Check sheet for the modelled part. Datum: model origin and axes. Units: mm. Face numbers are marked on the shaded views. A direction names the side the tool comes from. Coordinates: 2 decimals unless noted, no trailing zeros. Loops run counter-clockwise (first coordinate to the right, second up) from the corner with the lowest first, then second, coordinate; pieces in that order, holes last. Notation, with made-up numbers: (14, -9.5) -> (33, -9.5) arc R12 cw to (33, 7.5) -> close; hole circle Ø3 at (10.25, 54.5). An arc over 180 degrees is marked (long way). Use CSV: the item, a comma, the result in double quotes. Start each with the question number.
1. Sectioned sample at D-D, the plane y = -29. Record the cut outline in (x, z), and give its area (3 significant figures).
2. Sectioned sample at A-A, the plane z = 33. Record the cut outline in (x, y), and give its area (3 significant figures).
3. Set-up check for the marked faces 5, 6, 7 and 8: record each of +Z, -Z, +X, -X, +Y, -Y from which the full face is reachable in a straight line by a thin tool's end or side.
4. Release check for a two-part mould opening along X. For the marked faces 1, 2, 3 and 4 record: pulls with the +X half, pulls with the -X half, needs draft (parallel to the pull), parting line crosses it, or undercut.
5. Sectioned sample at C-C, the plane y = 0. Record the cut outline in (x, z).
6. Thickness scan on L1, parallel to Y at x = 10.5, z = 58; L2, parallel to Z at x = 53, y = -36.5; L3, parallel to Z at x = -14, y = -25.5. Record the ranges inside material, lowest first.
7. Gauge pin test, flat ends, axial feed: pin 1 (5 mm diameter, centred on x = -14.5, z = 63.5, fed in from +Y); pin 2 (16.5 mm diameter, centred on y = 27, z = 24.5, fed in from -X); pin 3 (6 mm diameter, centred on x = 31.5, z = 44.5, fed in from +Y); pin 4 (16 mm diameter, centred on x = 45.12, y = 0.47, fed in from +Z). Record the tip position at first contact, or that the pin passes through.
8. Sectioned sample at B-B, the plane x = 82. Record the cut outline in (y, z).
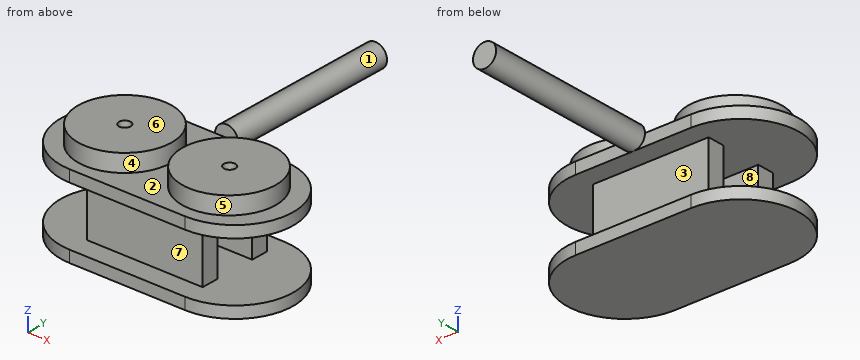
Autodesk Inventor part; units mm, degrees
ref_plane "YZ Plane" through (0, 0, 0) normal (1, 0, 0) x (0, 1, 0)
ref_plane "XZ Plane" through (0, 0, 0) normal (0, 1, 0) x (-1, 0, 0)
ref_plane "XY Plane" through (0, 0, 0) normal (0, 0, 1) x (1, 0, 0)
sketch "Sketch24" plane through (0, 0, 0) normal (0, 0, 1) x (1, 0, 0)
  line L0 (50, -50) -> (-50, -50)
  line L1 (-50, -50) -> (-50, 50)
  line L2 (-50, 50) -> (50, 50)
  line L3 (50, 50) -> (50, -50)
  line L4 (50, -50) -> (-50, 50) construction
  line L5 (-50, -50) -> (50, 50) construction
  circle A0 centre (50, 0) radius 50
  circle A1 centre (-50, 0) radius 50
  point P0 (0, 0)
  dimension "d55" = 100
  dimension "d56" = 100
  dimension "d57" = 100
  dimension "d58" = 100
extrude "Extrusion9" add sketch "Sketch24" along normal blind 10
sketch "Sketch25" plane through (0, 0, 10) normal (0, 0, 1) x (1, 0, 0)
  line L0 (50, 32.5) -> (-50, 32.5)
  line L1 (-50, 32.5) -> (-50, 17.5)
  line L2 (-50, 17.5) -> (50, 17.5)
  line L3 (50, 17.5) -> (50, 32.5)
  line L4 (50, 32.5) -> (-50, 17.5) construction
  line L5 (-50, 32.5) -> (50, 17.5) construction
  line L6 (50, -32.5) -> (-50, -32.5)
  line L7 (-50, -32.5) -> (-50, -17.5)
  line L8 (-50, -17.5) -> (50, -17.5)
  line L9 (50, -17.5) -> (50, -32.5)
  line L10 (50, -32.5) -> (-50, -17.5) construction
  line L11 (-50, -32.5) -> (50, -17.5) construction
  point P0 (0, 0)
  point P1 (0, 25)
  point P2 (0, -25)
  dimension "d61" = 100
  dimension "d62" = 15
  dimension "d63" = 15
extrude "Extrusion10" add sketch "Sketch25" along normal blind 50
sketch "Sketch38" plane through (0, 0, 60) normal (0, 0, 1) x (1, 0, 0)
  point P0 (0, 0)
sketch "Sketch39" plane through (0, 0, 10) normal (0, 0, 1) x (1, 0, 0)
  line L0 (-50, 17.5) -> (50, 17.5)
  point P0 (0, 0)
  dimension "d78" = 17.5
sketch "Sketch40" plane through (0, 0, 60) normal (0, 0, 1) x (1, 0, 0)
  line L0 (50, 50) -> (-50, 50)
  line L1 (-50, 50) -> (-50, -50)
  line L2 (-50, -50) -> (50, -50)
  line L3 (50, -50) -> (50, 50)
  line L4 (50, 50) -> (-50, -50) construction
  line L5 (-50, 50) -> (50, -50) construction
  circle A0 centre (50, 0) radius 50
  circle A1 centre (-50, 0) radius 50
  point P0 (0, 0)
  dimension "d79" = 100
  dimension "d80" = 100
  dimension "d81" = 100
  dimension "d82" = 100
extrude "Extrusion12" add sketch "Sketch40" along normal blind 10
sketch "Sketch43" plane through (0, 0, 70) normal (0, 0, 1) x (1, 0, 0)
  circle A0 centre (45, 0) radius 40
  circle A1 centre (-45, 0) radius 40
  point P0 (0, 0)
  dimension "d87" = 80
  dimension "d88" = 80
extrude "Extrusion13" add sketch "Sketch43" along normal blind 15
thread "Thread1"
thread "Thread2"
sketch "Sketch44" plane through (-45, 0, 85) normal (0, 0, 1) x (1, 0, 0)
  point P0 (45, 0)
  point P1 (0.1207, -0.2375)
hole "Hole1" at (-44.8793, -0.2375, 85) direction (0, 0, -1) diameter 10 depth 15
sketch "Sketch45" plane through (45, 0, 85) normal (0, 0, 1) x (1, 0, 0)
  point P0 (-45, 0)
  point P1 (0.1167, 0.4749)
hole "Hole2" at (45.1167, 0.4749, 85) direction (0, 0, -1) diameter 10 depth 15
sketch "Sketch49" plane through (0, 0, 70) normal (0, 0, 1) x (1, 0, 0)
  line L0 (-50, -50) -> (50, -50)
  line L1 (-4.7625, -50) -> (-4.7625, -90.4738)
  line L2 (5.1887, -50) -> (5.1887, -90.4738)
  line L3 (5.1887, -90.4738) -> (24.8137, -70.2369) construction
  line L4 (24.8137, -70.2369) -> (-4.7625, -90.4738) construction
  spline S0 degree 2 poles (5.1887, -90.4738) (24.8137, -70.2369) (-4.7625, -90.4738) knots 1 1 1 2 2 2
  point P0 (0, 0)
sketch "Sketch50" plane through (-50, 50, 60) normal (0, 1, 0) x (1, 0, 0)
  line L0 (0, -10) -> (100, -10)
  circle A0 centre (50, -10) radius 10
  point P0 (50, 60)
  dimension "d110" = 20
extrude "Extrusion14" add sketch "Sketch50" along normal blind 150
properties part number "base"
Completed:
1,outline,"(-90.73, 0) -> (90.73, 0) -> (90.73, 10) -> (50, 10) -> (50, 60) -> (90.73, 60) -> (90.73, 70) -> (72.55, 70) -> (72.55, 85) -> (17.45, 85) -> (17.45, 70) -> (-17.45, 70) -> (-17.45, 85) -> (-72.55, 85) -> (-72.55, 70) -> (-90.73, 70) -> (-90.73, 60) -> (-50, 60) -> (-50, 10) -> (-90.73, 10) -> close"
1,area,"10,300 mm²"
2,outline,"(-50, -32.5) -> (50, -32.5) -> (50, -17.5) -> (-50, -17.5) -> close; (-50, 17.5) -> (50, 17.5) -> (50, 32.5) -> (-50, 32.5) -> close"
2,area,"3,000 mm²"
3,face 5,"+Z"
3,face 6,"+Z, +X, -X, +Y, -Y"
3,face 7,"+X, -X, -Y"
3,face 8,"+X, -X"
4,face 1,"parting line crosses it"
4,face 2,"undercut"
4,face 3,"needs draft"
4,face 4,"undercut"
5,outline,"(-100, 0) -> (100, 0) -> (100, 10) -> (-100, 10) -> close; (-100, 60) -> (100, 60) -> (100, 70) -> (85, 70) -> (85, 85) -> (50.09, 85) -> (50.09, 70) -> (40.14, 70) -> (40.14, 85) -> (5, 85) -> (5, 70) -> (-5, 70) -> (-5, 85) -> (-39.88, 85) -> (-39.88, 70) -> (-49.87, 70) -> (-49.87, 85) -> (-85, 85) -> (-85, 70) -> (-100, 70) -> close"
6,L1,"-32.5 to -17.5, 17.5 to 32.5"
6,L2,"0 to 10, 60 to 85"
6,L3,"0 to 70"
7,pin 1,"y = 50"
7,pin 2,"x = -50"
7,pin 3,"y = 32.5"
7,pin 4,"z = 85"
8,outline,"(-38.42, 0) -> (38.42, 0) -> (38.42, 10) -> (-38.42, 10) -> close; (-38.42, 60) -> (38.42, 60) -> (38.42, 70) -> (15.2, 70) -> (15.2, 85) -> (-15.2, 85) -> (-15.2, 70) -> (-38.42, 70) -> close"
